from build123d import *

# Parameters (mm, degrees)
SKETCH1_R           = 2.6
SKETCH1_R_2         = 2.15
SKETCH1_R_3         = 2.1
BOSS_EXTRUDE1_DEPTH = 10
FILLET1_R           = 5
FILLET2_R           = 6
FILLET3_R           = 10
FILLET4_R           = 20
FILLET5_R           = 10
SKETCH2_R           = 1.65
CUT_EXTRUDE1_DEPTH  = 10


with BuildPart() as part:
    # Sketch1 → Boss-Extrude1 (new body)
    with BuildSketch(Plane(origin=(0, 0, 0), x_dir=(1, 0, 0), z_dir=(0, 1, 0))):
        Polygon((159.965380006, 15), (134.965380006, 28), (18, 28), (8, 33), (-2, 33), (-18, 16), (-18, 0), (0, 0), (129.965380006, 0), (159.965380006, 3), align=None)
        with Locations(Location((-11, 10, 0), (0, 0, 270))):
            Circle(SKETCH1_R, mode=Mode.SUBTRACT)
        with Locations(Location((129, 13, 0), (0, 0, 270))):
            Circle(SKETCH1_R_2, mode=Mode.SUBTRACT)
        with Locations(Location((154.965380006, 10, 0), (0, 0, 270))):
            Circle(SKETCH1_R, mode=Mode.SUBTRACT)
        with Locations(Location((1, 26, 0), (0, 0, 270))):
            Circle(SKETCH1_R, mode=Mode.SUBTRACT)
        with Locations(Location((50, 13, 0), (0, 0, 270))):
            Circle(SKETCH1_R_3, mode=Mode.SUBTRACT)
        with Locations(Location((70, 13, 0), (0, 0, 270))):
            Circle(SKETCH1_R_3, mode=Mode.SUBTRACT)
    extrude(amount=BOSS_EXTRUDE1_DEPTH)

    # Fillet1
    fillet1_edges = [part.edges().sort_by_distance(p)[0] for p in [
        (-18, 5, 0),
    ]]
    fillet(fillet1_edges, radius=FILLET1_R)

    # Fillet2
    # the kernel refuses this fillet: 6 mm, written as the material it takes off along each edge
    with BuildSketch(Plane(origin=(159.965380006, -9.106803364, -15), x_dir=(0, 0, 1), z_dir=(0, 1, 0))) as fillet2_piece_1:
        with BuildLine():
            CenterArc((FILLET2_R * 0.607120224288, -FILLET2_R), FILLET2_R, 90, 62.525568374)
            Line((-FILLET2_R * 0.280096576946, -FILLET2_R * 0.538647263358), (0, 0))
            Line((0, 0), (FILLET2_R * 0.607120224288, 0))
        make_face()
    extrude(amount=28.213606729, mode=Mode.SUBTRACT)
    with BuildSketch(Plane(origin=(159.965380006, -13.574813432, -3), x_dir=(-0.9950371902099892, 0, 0.0995037190209987), z_dir=(0, 1, 0))) as fillet2_piece_2:
        with BuildLine():
            CenterArc((FILLET2_R * 0.904987562112, -FILLET2_R), FILLET2_R, 90, 84.289406863)
            Line((-FILLET2_R * 0.0900496280979, -FILLET2_R * 0.900496280979), (0, 0))
            Line((0, 0), (FILLET2_R * 0.904987562112, 0))
        make_face()
    extrude(amount=37.149626863, mode=Mode.SUBTRACT)
    with BuildSketch(Plane(origin=(129.965380006, -0.748134317, 0), x_dir=(-1, 0, 0), z_dir=(0, 1, 0))) as fillet2_piece_3:
        with BuildLine():
            CenterArc((FILLET2_R * 0.0498756211209, -FILLET2_R), FILLET2_R, 90, 5.710593137)
            Line((-FILLET2_R * 0.0496280979001, -FILLET2_R * 0.00496280979001), (0, 0))
            Line((0, 0), (FILLET2_R * 0.0498756211209, 0))
        make_face()
    extrude(amount=11.496268634, mode=Mode.SUBTRACT)

    # Fillet3
    fillet3_edges = [part.edges().sort_by_distance(p)[0] for p in [
        (-18, 5, -16),
        (-2, 5, -33),
    ]]
    fillet(fillet3_edges, radius=FILLET3_R)

    # Fillet4
    fillet4_edges = [part.edges().sort_by_distance(p)[0] for p in [
        (134.965380006, 5, -28),
    ]]
    fillet(fillet4_edges, radius=FILLET4_R)

    # Fillet5
    fillet5_edges = [part.edges().sort_by_distance(p)[0] for p in [
        (8, 5, -33),
        (18, 5, -28),
    ]]
    fillet(fillet5_edges, radius=FILLET5_R)

    # Sketch2 → Cut-Extrude1 (cut)
    with BuildSketch(Plane.XY):
        with Locations((47, 5)):
            Circle(SKETCH2_R)
        with Locations((108, 5)):
            Circle(SKETCH2_R)
    extrude(amount=-CUT_EXTRUDE1_DEPTH, mode=Mode.SUBTRACT)


solid = part.part
CAD build for the part. Positions are in the model's coordinates, mm. A direction names the side the tool comes from. Give positions to 0.01 mm unless a question says otherwise; leave off trailing zeros. Order: outer loops, then holes, each group sorted by start corner. A loop starts at its lowest first (then second) coordinate and runs counter-clockwise, first axis right, second up. Notation, with made-up numbers: (84, 50) -> (92, 50) arc R20 cw to (92, 60) -> close; hole circle Ø5 at (-19.5, -38.75). An arc over 180 degrees is marked (long way). Return JSON: item names as keys, results as strings.
Q1. Saw through at C-C (z = -21). Write the cut outline in (x, y).
Working result:
{"outline": "(-13.29, 0) -> (148.43, 0) -> (148.43, 10) -> (-13.29, 10) -> close"}
Q2. Which spindle directions (+Z, -Z, +X, -X, +Y, -Y) get a long thin tool onto all of the face, cutting with end or side? Do faces 1 (the face through (108, 5, -10)), 2 (the face through (76, 5, -28)), 3 (the face through (70, 0, -17)). Say none if no direction does.
Working result:
{"face 1": "+Z", "face 2": "-Z, +X, +Y, -Y", "face 3": "+Z, -Z, +X, -X, -Y"}
Q3. Drill centre lines: line 1 (X direction, y = 8.75, z = -10); line 2 (X direction, y = 7, z = -13); line 3 (Z direction, x = 129, y = 6.5). Where is each one in solid material? Low to high.
Working result:
{"line 1": "-18 to -13.6, -8.4 to 152.37, 157.57 to 159.97", "line 2": "-17.95 to 47.9, 52.1 to 67.9, 72.1 to 126.85, 131.15 to 159.74", "line 3": "-28 to -15.15, -10.85 to 0"}
Q4. Mould opens along Z. For faces 4 (the face through (-10.049, 4.93, -24.448)), 5 (the face through (-1.54, 4.93, -26.56)), 6 (the face through (142.243, 4.93, -1.228)) say: pulls with the +Z half, pulls with the -Z half, needs draft (parallel to the pull), parting line crosses it, or undercut.
Working result:
{"face 4": "pulls with the -Z half", "face 5": "undercut", "face 6": "pulls with the +Z half"}
Q5. Saw through at B-B (x = -11). Write the cut outline in (y, z), then the cut area to 3 significant figures.
Working result:
{"outline": "(0, -23.44) -> (10, -23.44) -> (10, -12.6) -> (0, -12.6) -> close; (0, -7.4) -> (10, -7.4) -> (10, 0) -> (0, 0) -> close", "area": "182 mm²"}
Q6. Saw through at A-A (x = 108). Write the cut outline in (y, z).
Working result:
{"outline": "(0, -28) -> (10, -28) -> (10, 0) -> (6.65, 0) -> (6.65, -10) -> (3.35, -10) -> (3.35, 0) -> (0, 0) -> close"}
Q7. Flat gauge pins, fed straight in: pin 1 (7 mm diameter, centred on x = -11, z = -10, fed in from -Y); pin 2 (2 mm diameter, centred on y = 8.5, z = -29, fed in from -X); pin 3 (2.5 mm diameter, centred on x = 47, y = 5, fed in from -Z); pin 4 (1.5 mm diameter, centred on x = 8.5, y = 7, fed in from -Z). Where does each tip first touch, or does it go through?
Working result:
{"pin 1": "y = 0", "pin 2": "x = -6.71", "pin 3": "z = -28", "pin 4": "z = -32.77"}
